Can you work these out from the drawing? Everything is in mm from the part's minimum corner. Round coordinates to 2 decimals unless told otherwise and drop trailing zeros. Loops run counter-clockwise (first coordinate to the right, second up) from the corner with the lowest first, then second, coordinate; pieces in that order, holes last. Notation, with made-up numbers: (3, 12) -> (19, 12) arc R17 ccw to (19, 41) -> close; hole circle Ø9 at (63.5, 87). An arc over 180 degrees is marked (long way). One line per item, written item: value.
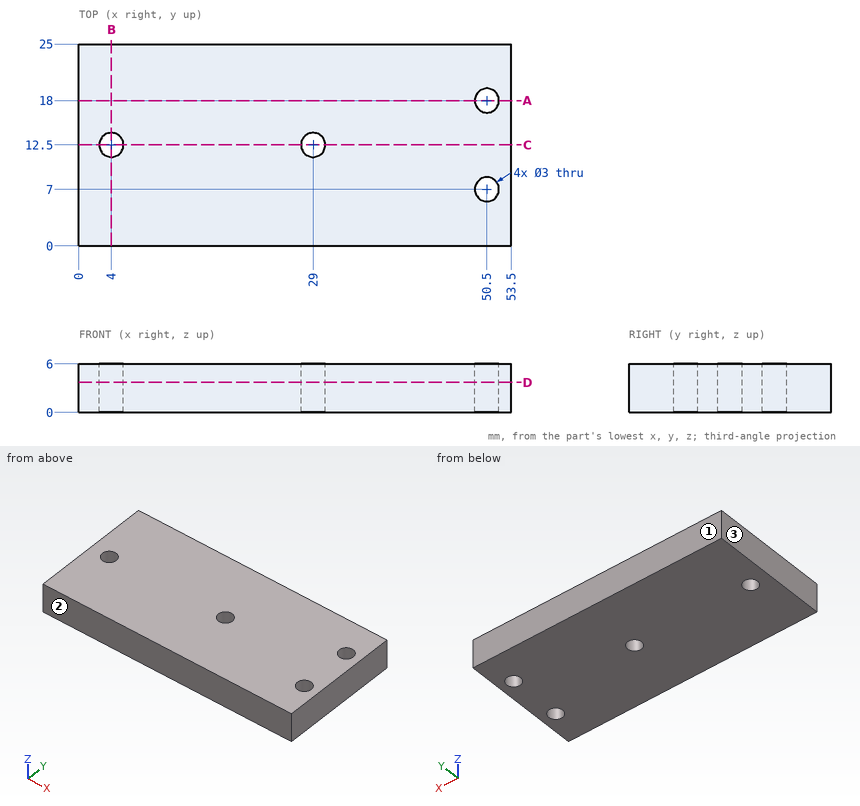
(1) Please list where these lines run through material, in increasing order: L1, parallel to X at y = 12.5, z = 1.8; L2, parallel to Y at x = 50.5, z = 1.55; L3, parallel to X at y = 12, z = 4.1.
Results below:
L1: x = 0 to 2.5, 5.5 to 27.5, 30.5 to 53.5
L2: y = 0 to 5.5, 8.5 to 16.5, 19.5 to 25
L3: x = 0 to 2.59, 5.41 to 27.59, 30.41 to 53.5
(2) Imagine slicing it at A-A on y = 18. Write out the boundary of the cut face in (x, z).
Results below:
outline: (0, 0) -> (49, 0) -> (49, 6) -> (0, 6) -> close; (52, 0) -> (53.5, 0) -> (53.5, 6) -> (52, 6) -> close
(3) We'd pull the mould along Y, two halves only. Please class the marked faces 1, 2 and 3: +Y half, -Y half, draft (parallel to the pull), parting line (faces both ways), or undercut.
Results below:
face 1: +Y half
face 2: -Y half
face 3: draft
(4) Imagine slicing it at B-B on x = 4. Write out the boundary of the cut face in (y, z), then the cut area to 3 significant figures.
Results below:
outline: (0, 0) -> (11, 0) -> (11, 6) -> (0, 6) -> close; (14, 0) -> (25, 0) -> (25, 6) -> (14, 6) -> close
area: 132 mm²
(5) Imagine slicing it at C-C on y = 12.5. Write out the boundary of the cut face in (x, z).
Results below:
outline: (0, 0) -> (2.5, 0) -> (2.5, 6) -> (0, 6) -> close; (5.5, 0) -> (27.5, 0) -> (27.5, 6) -> (5.5, 6) -> close; (30.5, 0) -> (53.5, 0) -> (53.5, 6) -> (30.5, 6) -> close
(6) Imagine slicing it at D-D on z = 3.7. Write out the boundary of the cut face in (x, y), then the cut area to 3 significant figures.
Results below:
outline: (0, 0) -> (53.5, 0) -> (53.5, 25) -> (0, 25) -> close; hole circle Ø3 at (4, 12.5); hole circle Ø3 at (29, 12.5); hole circle Ø3 at (50.5, 7); hole circle Ø3 at (50.5, 18)
area: 1,310 mm²
